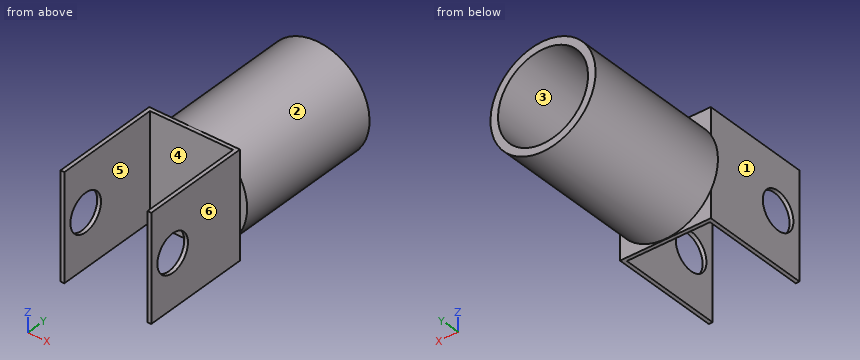
```python
from build123d import *

# Parameters (mm, degrees)
SKETCH1_R               = 69.5
SKETCH1_R_2             = 59.5
BOSS_EXTRUDE1_DEPTH     = 200
SKETCH2_W               = 120
SKETCH2_H               = 140
BOSS_EXTRUDE2_DEPTH     = 5
SKETCH3_W               = 5
SKETCH3_H               = 140
BOSS_EXTRUDE3_DEPTH     = 140
CUT_EXTRUDE1_DEPTH      = 249.334955252
CUT_EXTRUDE1_DEPTH_BACK = 249.334955252
SKETCH4_R               = 25


with BuildPart() as part:
    # Sketch1 → Boss-Extrude1 (new body)
    with BuildSketch(Plane(origin=(0, 0, 0), x_dir=(1, 0, 0), z_dir=(0, 1, 0))):
        with Locations(Location((0, 0, 0), (0, 0, 270))):
            Circle(SKETCH1_R)
        with Locations(Location((0, 0, 0), (0, 0, 270))):
            Circle(SKETCH1_R_2, mode=Mode.SUBTRACT)
    extrude(amount=BOSS_EXTRUDE1_DEPTH)

    # Sketch2 → Boss-Extrude2 (add)
    with BuildSketch(Plane.XZ):
        Rectangle(SKETCH2_W, SKETCH2_H)
    extrude(amount=BOSS_EXTRUDE2_DEPTH)

    # Sketch3 → Boss-Extrude3 (add)
    with BuildSketch(Plane.XZ.offset(5)):
        with Locations((-57.5, 0)):
            Rectangle(SKETCH3_W, SKETCH3_H)
        with Locations((57.5, 0)):
            Rectangle(SKETCH3_W, SKETCH3_H)
    extrude(amount=BOSS_EXTRUDE3_DEPTH)

    # Sketch4 → Cut-Extrude1 (cut, two sides: drawn at the far end of the back side and taken through both)
    with BuildSketch(Plane.ZY.offset(60).offset(-CUT_EXTRUDE1_DEPTH_BACK)):
        with Locations((0, -110)):
            Circle(SKETCH4_R)
    extrude(amount=CUT_EXTRUDE1_DEPTH + CUT_EXTRUDE1_DEPTH_BACK, mode=Mode.SUBTRACT)


solid = part.part
```
Geometry check sheet. Reference: the model listing, model coordinates, mm. Face numbers are marked on the shaded views. A direction names the side the tool comes from. Give positions to 0.01 mm unless a question says otherwise; leave off trailing zeros. Order: outer loops, then holes, each group sorted by start corner. A loop starts at its lowest first (then second) coordinate and runs counter-clockwise, first axis right, second up. Notation, with made-up numbers: (1.5, 59) - (20.5, 59) arc R21 ccw to (20.5, 82) - close; hole circle Ø3 at (60, 72.5). An arc over 180 degrees is marked (long way). Write item = value, one per line. Start each with the question number.
1) Section check D-D (x = 0). Enter the section's corners in (y, z), then the cut area to 3 significant figures.
2) Section check C-C (y = -110). Enter the section's corners in (x, z), then the cut area to 3 significant figures.
3) Scan lines: L1, parallel to Y at x = -56.9, z = 0; L2, parallel to X at y = -83.5, z = 33; L3, parallel to X at y = 128, z = 0. Record each from-to range of solid material in increasing order.
4) Draft check along X on the marked faces 1, 2, 3 and 4. Enter one of: released by +X, released by -X, zero draft, split by the parting line, or undercut.
5) Section check A-A (y = -50.5). Enter the section's corners in (x, z), then the cut area to 3 significant figures.
6) Access from +Z, -Z, +X, -X, +Y, -Y to the whole of each face (thin tool, end or side, straight path). Record for the marked faces 5 and 6.
7) Section check B-B (z = 0). Enter the section's corners in (x, y), then the cut area to 3 significant figures.
8) Gauge pin test, flat ends, axial feed: pin 1 Ø8 at (x, z) = (-16, -46.5) entering from +Y; pin 2 Ø4 at (x, y) = (-45.5, 108) entering from +Z; pin 3 Ø6 at (y, z) = (157.5, -17) entering from -X. Record the tip position at first contact, or that the pin passes through.
Geometry check:
q1.outline = (-5, -70) - (0, -70) - (0, -69.5) - (200, -69.5) - (200, -59.5) - (0, -59.5) - (0, 59.5) - (200, 59.5) - (200, 69.5) - (0, 69.5) - (0, 70) - (-5, 70) - close
q1.area = 4,700 mm2
q2.outline = (-60, -70) - (-55, -70) - (-55, -25) - (-60, -25) - close; (-60, 25) - (-55, 25) - (-55, 70) - (-60, 70) - close; (55, -70) - (60, -70) - (60, -25) - (55, -25) - close; (55, 25) - (60, 25) - (60, 70) - (55, 70) - close
q2.area = 900 mm2
q3.L1 = -145 to -135, -85 to 0
q3.L2 = -60 to -55, 55 to 60
q3.L3 = -69.5 to -59.5, 59.5 to 69.5
q4.face_1 = released by -X
q4.face_2 = split by the parting line
q4.face_3 = undercut
q4.face_4 = undercut
q5.outline = (-60, -70) - (-55, -70) - (-55, 70) - (-60, 70) - close; (55, -70) - (60, -70) - (60, 70) - (55, 70) - close
q5.area = 1,400 mm2
q6.face_5 = +Z, -Z, -Y
q6.face_6 = +Z, -Z, +X, -Y
q7.outline = (-69.5, 0) - (-60, 0) - (-60, -85) - (-55, -85) - (-55, -5) - (55, -5) - (55, -85) - (60, -85) - (60, 0) - (69.5, 0) - (69.5, 200) - (59.5, 200) - (59.5, 0) - (-59.5, 0) - (-59.5, 200) - (-69.5, 200) - close; (-60, -145) - (-55, -145) - (-55, -135) - (-60, -135) - close; (55, -145) - (60, -145) - (60, -135) - (55, -135) - close
q7.area = 5,500 mm2
q8.pin_1 = 0
q8.pin_2 = 54.2
q8.pin_3 = -68.08
